```python
from build123d import *

# Parameters (mm, degrees)
F0_W      = 279.4
F0_H      = 101.6
F1_DEPTH  = 3.175
F2_W      = 25.4
F2_H      = 44.45
F2_H_2    = 31.75
F3_DEPTH  = 3.176
F4_W      = 12.192
F4_H      = 21.082
F5_DEPTH  = 3.175
F7_D      = 6.6
F9_D      = 13.2
F11_D     = 13.2
F13_D     = 6.6
F14_W     = 25.4
F14_H     = 3.175
F15_DEPTH = 25.4
F17_D     = 6.6
F19_D     = 9
F20_D     = 6.6


with BuildPart() as f1:
    # F0 (on Top) → F1 (new body)
    with BuildSketch(Plane.XY):
        with Locations((37.6198536942, 37.7514991719)):
            Rectangle(F0_W, F0_H)
    extrude(amount=F1_DEPTH)

    # F2 (on face) → F3 (cut, through all)
    with BuildSketch(Plane.XY.offset(3.175)):
        with Locations((-89.3801463058, 9.1764991719)):
            Rectangle(F2_W, F2_H)
        with Locations((-89.3801463058, 72.6764991719)):
            Rectangle(F2_W, F2_H_2)
    extrude(amount=-F3_DEPTH, mode=Mode.SUBTRACT)

    # F4 (on face) → F5 (join)
    with BuildSketch(Plane(origin=(0, 0, 0), x_dir=(1, 0, 0), z_dir=(0, 0, -1))):
        with Locations((-23.0861463058, 23.5895008281)):
            Rectangle(F4_W, F4_H)
        Polygon((-16.9901463058, 13.0485008281), (-29.1821463058, 13.0485008281), (-76.6801463058, 13.0485008281), (-76.6801463058, -31.4014991719), (-102.0801463058, -31.4014991719), (-102.0801463058, -56.8014991719), (-76.6801463058, -56.8014991719), (-76.6801463058, -88.5514991719), (177.3198536942, -88.5514991719), (177.3198536942, 13.0485008281), align=None)
    extrude(amount=-F5_DEPTH)

    # F7 (through all)
    with Locations(Plane.XY.offset(3.175)):
        with Locations((-89.3801463058, 44.1014991719)):
            Hole(F7_D / 2)

    # F9 (through all)
    with Locations(Plane.XY.offset(3.175)):
        with Locations((-63.9801463058, 75.8514991719)):
            Hole(F9_D / 2)

    # F11 (through all)
    with Locations(Plane.XY.offset(3.175)):
        with Locations((-63.9801463058, -0.3485008281), (164.6198536942, -0.3485008281), (164.6198536942, 75.8514991719)):
            Hole(F11_D / 2)

    # F13 (through all)
    with Locations(Plane.XY.offset(3.175)):
        with Locations((-23.0861463058, -24.7325008281)):
            Hole(F13_D / 2)

    # F14 (on face) → F15 (join)
    with BuildSketch(Plane.YZ.offset(177.3198536942)):
        with Locations((44.1014991719, 1.5875)):
            Rectangle(F14_W, F14_H)
    extrude(amount=F15_DEPTH)

    # F17 (through all)
    with Locations(Plane(origin=(0, 0, 0), x_dir=(1, 0, 0), z_dir=(0, 0, -1))):
        with Locations((190.0198536942, -44.1014991719)):
            Hole(F17_D / 2)

    # F19 (through all)
    with Locations(Plane.XY.offset(3.175)):
        with Locations((-32.2301463058, 59.8764993719), (9.0448536942, 59.8764993719), (50.3198536942, 59.8764993719), (91.5948536942, 59.8764993719), (132.8698536942, 59.8764993719), (132.8698536942, 15.6264989719), (91.5948536942, 15.6264989719), (50.3198536942, 15.6264989719), (9.0448536942, 15.6264989719), (-32.2301463058, 15.6264989719)):
            Hole(F19_D / 2)

    # F20 (through all)
    with Locations(Plane.XY.offset(3.175)):
        with Locations((-32.2301463058, 72.6764991719), (-32.2301463058, 2.8264991719), (9.0448536942, 2.8264991719), (9.0448536942, 72.6764991719), (50.3198536942, 72.6764991719), (50.3198536942, 2.8264991719), (91.5948536942, 2.8264991719), (91.5948536942, 72.6764991719), (132.8698536942, 72.6764991719), (132.8698536942, 2.8264991719)):
            Hole(F20_D / 2)


solid = f1.part
```
Input: part model. Units: mm. Frame: model coordinates. Coordinates: 2 decimals unless noted, no trailing zeros. Loops run counter-clockwise (first coordinate to the right, second up) from the corner with the lowest first, then second, coordinate; pieces in that order, holes last. Notation, with made-up numbers: M 15.5,-28.75 L 46.5,-28.75 A13 cw 46.5,-23.75 Z; hole C 85,34 d9. An arc over 180 degrees is marked long. One line per item, written item: value.
(1) Line query: line 1 along Y through (x, z) = (91, 1.25); line 2 along X through (y, z) = (58, 0.55); line 3 along X through (y, z) = (-3, 1.75). Output: solid intervals per line, ascending. Write a range as from..to.
Filled in:
line 1: -13.05..-0.42, 6.07..11.17, 20.09..55.42, 64.34..69.43, 75.92..88.55
line 2: -76.68..-36.32, -28.14..4.95, 13.13..46.23, 54.41..87.5, 95.68..128.78, 136.96..177.32
line 3: -76.68..-70.02, -57.94..158.58, 170.66..177.32
(2) Section C-C (z = 1.2). Give the number of separate pieces and of enclosed holes in the cut face, and give its area (3 significant figures).
Filled in:
separate pieces: 1
enclosed holes: 27
area: 25,700 mm^2
(3) Pin query (flat end, axial travel): pin 1 (7.5 mm diameter, centred on x = 50.32, y = 2.83, fed in from -Z); pin 2 (1.6 mm diameter, centred on x = 67, z = 1, fed in from -Y); pin 3 (1.5 mm diameter, centred on y = 16.5, z = 0.5, fed in from -X); pin 4 (1.6 mm diameter, centred on y = 69, z = 1, fed in from +X). Return the tip coordinate at first contact, or that it passes through.
Filled in:
pin 1: z = 0
pin 2: y = -13.05
pin 3: x = -76.68
pin 4: x = 177.32
(4) Section A-A (x = 168). Output: boundary loops of the cut face in (y, z) (1 decimal), and give its area (3 significant figures).
Filled in:
outline: M -13,0 L -6,0 L -6,3.2 L -13,3.2 Z; M 5.3,0 L 70.2,0 L 70.2,3.2 L 5.3,3.2 Z; M 81.5,0 L 88.6,0 L 88.6,3.2 L 81.5,3.2 Z
area: 251 mm^2
(5) Section B-B (x = 35.5). Output: boundary loops of the cut face in (y, z) (1 decimal), and give its area (3 significant figures).
Filled in:
outline: M -13,0 L 88.6,0 L 88.6,3.2 L -13,3.2 Z
area: 323 mm^2
(6) Pull-direction query (X, two-part tool) for faces 1 (the cylindrical face through (131.1, 75.46, 1.57)), 2 (the flat face through (48, 40, 0)); classes: +X half, -X half, draft (parallel to the pull), parting line (faces both ways), or undercut.
Filled in:
face 1: undercut
face 2: draft
